CAD build for the part. Positions are in the model's coordinates, mm. A direction names the side the tool comes from. Round coordinates to 2 decimals unless told otherwise and drop trailing zeros. Write each loop counter-clockwise with the first axis right and the second up, starting at its lowest first coordinate (ties: lowest second). Pieces come first, ordered by that corner, then holes. Notation, with made-up numbers: (51, 16) - (68, 16) arc R25 cw to (68, 47) - close; hole circle Ø2 at (75, 13). An arc over 180 degrees is marked (long way). Answer in a Markdown table with one row per item.
Autodesk Inventor part; units mm, degrees
ref_plane "YZ Plane" through (0, 0, 0) normal (1, 0, 0) x (0, 1, 0)
ref_plane "XZ Plane" through (0, 0, 0) normal (0, 1, 0) x (-1, 0, 0)
ref_plane "XY Plane" through (0, 0, 0) normal (0, 0, 1) x (1, 0, 0)
sketch "Sketch1" plane through (0, 0, 0) normal (0, 1, 0) x (-1, 0, 0)
  arc A0 (8, 6) -> (8, -6) centre (0, 0) ccw
  arc A1 (7, 5.6569) -> (7, -5.6569) centre (0, 0) ccw
  line L0 (8, 0) -> (8, -6)
  line L1 (8, 6) -> (8, 0)
  line L2 (7, -5.6569) -> (7, 5.6569)
  dimension "d0" = 20
  dimension "d1" = 1
extrude "Extrusion1" add sketch "Sketch1" along normal blind 8
sketch "Sketch2" plane through (0, 0, 0) normal (0, -1, 0) x (1, 0, 0)
  point P0 (0, 0)
sketch "Sketch3" plane through (-8, 0, -6) normal (-1, 0, 0) x (0, 0, 1)
  line L0 (0, 8) -> (12, 8) construction
  line L1 (6, 8) -> (6, -6) construction
  circle A0 centre (6, -6) radius 14
  point P0 (6, 0)
  dimension "d7" = 14
sketch "Sketch4" plane through (0, 8, 0) normal (0, 1, 0) x (1, 0, 0)
  circle A0 centre (0, 0) radius 10
  circle A1 centre (0, 0) radius 9
extrude "Extrusion2" add sketch "Sketch4" against normal blind 8
extrude "Extrusion3" cut sketch "Sketch3" along normal blind 8
sketch "Sketch5" plane through (0, 8, 0) normal (0, 1, 0) x (1, 0, 0)
  circle A0 centre (0, 0) radius 10
  circle A1 centre (0, 0) radius 9
extrude "Extrusion4" add sketch "Sketch5" along normal blind 7
sketch "Sketch6" plane through (0, 15, 0) normal (0, 1, 0) x (1, 0, 0)
  circle A0 centre (0, 0) radius 9
  arc A1 (-7, -5.6569) -> (-7, 5.6569) centre (0, 0) ccw
  circle A2 centre (0, 0) radius 8
  dimension "d14" = 16
extrude "Extrusion5" add sketch "Sketch6" against normal up to surface (7 mm away)
sketch "Sketch7" plane through (0, 8, 0) normal (0, -1, 0) x (1, 0, 0)
  arc A0 (-8, 4.1231) -> (-9, 0) centre (0, 0) ccw
  circle A1 centre (0, 0) radius 9
  circle A2 centre (0, 0) radius 8
  line L0 (-8, -4.1231) -> (-8, 0)
  line L1 (-8, 0) -> (-8, 4.1231)
  line L2 (-8, -4.1231) -> (-8, 4.1231)
  line L3 (-7, 5.6569) -> (-7, 3.873)
  line L4 (-7, -3.873) -> (-7, -5.6569)
  line L5 (-7, 5.6569) -> (-7, -5.6569)
extrude "Extrusion6" add sketch "Sketch7" along normal up to surface (8 mm away) contours A1 L4 A2 L3
sketch "Sketch8" plane through (0, 15, 0) normal (0, 1, 0) x (1, 0, 0)
  circle A0 centre (0, 0) radius 9
  circle A1 centre (0, 0) radius 8
  circle A2 centre (0, 0) radius 9
  dimension "d19" = 18
extrude "Extrusion7" add sketch "Sketch8" along normal blind 7
sketch "Sketch9" plane through (0, 22, 0) normal (0, 1, 0) x (1, 0, 0)
  circle A0 centre (0, 0) radius 8
  circle A1 centre (0, 0) radius 7
  dimension "d22" = 14
extrude "Extrusion8" add sketch "Sketch9" against normal up to surface (22 mm away)
sketch "Sketch10" plane through (0, 22, 0) normal (0, 1, 0) x (1, 0, 0)
  circle A0 centre (0, 0) radius 7
  circle A1 centre (0, 0) radius 7
  circle A2 centre (0, 0) radius 8
  dimension "d25" = 16
extrude "Extrusion9" add sketch "Sketch10" along normal blind 2.5
sketch "Sketch11" plane through (0, 24.5, 0) normal (0, 1, 0) x (1, 0, 0)
  circle A0 centre (0, 0) radius 8
  circle A1 centre (0, 0) radius 7
  circle A2 centre (0, 0) radius 7
extrude "Extrusion10" add sketch "Sketch11" against normal up to surface (24.5 mm away) contours A1
sketch "Sketch13" plane through (0, 0, 0) normal (0, 0, 1) x (1, 0, 0)
  line L0 (0, 24.5) -> (6.4, 24.5)
  line L1 (0, 24.5) -> (6.4, 24.5)
  line L2 (0, 26.5) -> (0, 24.5)
  arc A0 (6.4, 24.5) -> (0, 26.5) centre (0, 15.26) ccw
  line L3 (0, 0) -> (0, 24.5)
  line L4 (8, 24.5) -> (-8, 24.5)
revolve "Revolution1" add sketch "Sketch13" angle 360 about axis through (0, 26.5, 0) along (0, -1, 0)
properties part number "button 3"
Q1. Saw through at C-C on x = 2.5. List the corners of the cut face in (y, z), then the cut area to 3 significant figures.
Computed:
| item | result |
|---|---|
| outline | (0, -9.68) - (15, -9.68) - (15, -8.65) - (22, -8.65) - (22, -7.6) - (24.5, -7.6) - (24.5, -5.89) arc R10.96 ccw to (24.5, 5.89) - (24.5, 7.6) - (22, 7.6) - (22, 8.65) - (15, 8.65) - (15, 9.68) - (0, 9.68) - close |
| area | 463 mm2 |
Q2. Pull direction Z, two halves, no side cores. Call faces 4 (the flat face through (1, 0, 0)), 5 (the cylindrical face through (-1.73, 23.23, -7.81)), 6 (the cylindrical face through (-8.422, 7.849, -3.172)): released by +Z, released by -Z, zero draft, split by the parting line, or undercut.
Computed:
| item | result |
|---|---|
| face 4 | zero draft |
| face 5 | split by the parting line |
| face 6 | undercut |
Q3. Saw through at D-D on z = 3. List the corners of the cut face in (x, y), then the cut area to 3 significant figures.
Computed:
| item | result |
|---|---|
| outline | (-9.54, 7.67) - (-8.49, 7.67) - (-8.49, 8) - (-8, 8) - (-8, 0) - (9.54, 0) - (9.54, 15) - (8.49, 15) - (8.49, 22) - (7.42, 22) - (7.42, 24.5) - (5.65, 24.5) arc R10.83 ccw to (-5.65, 24.5) - (-7.42, 24.5) - (-7.42, 22) - (-8.49, 22) - (-8.49, 15) - (-9.54, 15) - close |
| area | 442 mm2 |
Q4. Saw through at B-B on z = -8.5. List the corners of the cut face in (x, y), then the cut area to 3 significant figures.
Computed:
| item | result |
|---|---|
| outline | (-5.27, 0) - (5.27, 0) - (5.27, 15) - (2.96, 15) - (2.96, 22) - (-2.96, 22) - (-2.96, 15) - (-5.27, 15) - close |
| area | 199 mm2 |
Q5. Saw through at A-A on x = 0. List the corners of the cut face in (y, z), then the cut area to 3 significant figures.
Computed:
| item | result |
|---|---|
| outline | (0, -10) - (15, -10) - (15, -9) - (22, -9) - (22, -8) - (24.5, -8) - (24.5, -6.4) arc R11.24 ccw to (24.5, 6.4) - (24.5, 8) - (22, 8) - (22, 9) - (15, 9) - (15, 10) - (0, 10) - close |
| area | 483 mm2 |
Q6. Drill centre lines: line 1 (Y direction, x = -3.5, z = 7.25); line 2 (Y direction, x = 7.5, z = 5.5); line 3 (X direction, y = 4, z = 3). Where is each one in solid material? Low to high.
Computed:
| item | result |
|---|---|
| line 1 | y = 0 to 22 |
| line 2 | y = 0 to 15 |
| line 3 | x = -8 to 9.54 |
Q7. 3-axis set-ups, long thin cutter, end or side, ignore diameter. For faces 1 (the flat face through (-8.4, 8, -0.1)), 2 (the flat face through (0, 24.5, -7)), 3 (the cylindrical face through (-9.2, 8, -0.1)): which of +Z, -Z, +X, -X, +Y, -Y reach the whole face in a straight line?
Computed:
| item | result |
|---|---|
| face 1 | -Y |
| face 2 | +Y |
| face 3 | -X, -Y |
Q8. Flat gauge pins, fed straight in: pin 1 (6 mm diameter, centred on x = 4.5, z = 0, fed in from +Y); pin 2 (1 mm diameter, centred on x = 5.5, y = 17, fed in from -Z); pin 3 (6 mm diameter, centred on y = 21, z = -4, fed in from +X). Where does each tip first touch, or does it go through?
Computed:
| item | result |
|---|---|
| pin 1 | stops at y = 26.4 |
| pin 2 | stops at z = -7.48 |
| pin 3 | stops at x = 8.94 |
